Geometry check sheet. Reference: the model listing, model coordinates, mm. A direction names the side the tool comes from. Give positions to 0.01 mm unless a question says otherwise; leave off trailing zeros. Write each loop counter-clockwise with the first axis right and the second up, starting at its lowest first coordinate (ties: lowest second). Pieces come first, ordered by that corner, then holes. Notation, with made-up numbers: (85.25, -27.5) - (134.25, -27.5) arc R24 ccw to (134.25, -4.5) - close; hole circle Ø6 at (36, 1). An arc over 180 degrees is marked (long way). Write item = value, one per line. Start each with the question number.
(1) Section check B-B, the plane x = 0. Enter the section's corners in (y, z).
(2) Section check A-A, the plane y = 0. Enter the section's corners in (x, z), plus the area to 3 significant figures.
(3) Access from +Z, -Z, +X, -X, +Y, -Y to the whole of each face (thin tool, end or side, straight path). Record for faces 1 (the cylindrical face through (15.48, 11.37, 4.44)), 2 (the flat face through (24.21, -6.415, 4.437)).
(4) Section check C-C, the plane z = 5.5. Enter the section's corners in (x, y), plus the area to 3 significant figures.
(5) Draft check along Y on faces 3 (the flat face through (16, -5.139, 4)), 4 (the cylindrical face through (14.09, 7.79, 4.44)), 5 (the cylindrical face through (14.09, 2.65, 4.56)), 6 (the flat face through (15, 0, 9)). Enter one of: pulls with the +Y half, pulls with the -Y half, needs draft (parallel to the pull), parting line crosses it, or undercut.
(6) Depth check by flat-ended pin: pin 1 Ø2 at (y, z) = (6.5, 7) entering from -X; pin 2 Ø1.8 at (x, y) = (15.59, 2.59) entering from -Z; pin 3 Ø4 at (x, z) = (8.5, 2.5) entering from +Y; pin 4 Ø2 at (y, z) = (-2.5, 1) entering from +X. Enter the tip coordinate at first touch or a pass-through.
(7) Thickness scan on L1, parallel to Y at x = 0, z = 2.75; L2, parallel to X at y = 1.75, z = 6; L3, parallel to Y at x = 12.5, z = 1.25. Record the ranges inside material, lowest first.
(8) Section check D-D, the plane y = 8.5. Enter the section's corners in (x, z).
Autodesk Inventor part; units mm, degrees
ref_plane "YZ Plane" through (0, 0, 0) normal (1, 0, 0) x (0, 1, 0)
ref_plane "XZ Plane" through (0, 0, 0) normal (0, 1, 0) x (-1, 0, 0)
ref_plane "XY Plane" through (0, 0, 0) normal (0, 0, 1) x (1, 0, 0)
sketch "Sketch1" plane through (0, 0, 0) normal (0, 0, 1) x (1, 0, 0)
  line L0 (19.4476, -5.1392) -> (29.1069, -7.7274)
  line L1 (19.4476, -5.1392) -> (23.5887, 10.3156) construction
  line L2 (11.7298, -5.1392) -> (19.4476, -5.1392)
  line L3 (7.5887, 10.3156) -> (11.7298, -5.1392) construction
  line L4 (7.5887, 10.3156) -> (23.5887, 10.3156) construction
  arc A0 (23.5887, 10.3156) -> (7.5887, 10.3156) centre (15.5887, -19.5408) ccw
  line L5 (11.7298, -5.1392) -> (2.0706, -7.7274)
  line L6 (-2.0706, 7.7274) -> (7.5887, 10.3156)
  arc A1 (-2.0706, 7.7274) -> (2.0706, -7.7274) centre (0, 0) ccw
  circle A2 centre (0, 0) radius 8 construction
  circle A3 centre (31.1774, 0) radius 8 construction
  arc A4 (29.1069, -7.7274) -> (33.248, 7.7274) centre (31.1774, 0) ccw
  line L7 (23.5887, 10.3156) -> (33.248, 7.7274)
  circle A5 centre (0, 0) radius 1.5
  circle A6 centre (31.1774, 0) radius 1.5
  circle A7 centre (15.5887, 7.8608) radius 1.5
  point P0 (0, 0)
  point P1 (15.5887, 10.3156)
  dimension "d0" = 16
  dimension "d1" = 16
  dimension "d2" = 16
  dimension "d3" = 10
  dimension "d4" = 10
  dimension "d5" = 16
  dimension "d6" = 16
  dimension "d7" = 75
  dimension "d8" = 3
  dimension "d9" = 3
  dimension "d10" = 3
  dimension "d11" = 13
extrude "Extrusion1" add sketch "Sketch1" along normal blind 9
sketch "Sketch3" plane through (0, 0, 9) normal (0, 0, 1) x (1, 0, 0)
  circle A0 centre (15.5887, 2.5882) radius 1.5
  line L0 (11.7298, -5.1392) -> (19.4476, -5.1392) construction
  line L1 (7.5887, 10.3156) -> (-2.0706, 7.7274) construction
  line L2 (33.248, 7.7274) -> (23.5887, 10.3156) construction
  line L3 (7.5887, 10.3156) -> (23.5887, 10.3156) construction
  line L4 (15.5887, 10.3156) -> (15.5887, -5.1392) construction
  point P0 (0, 0)
  point P1 (15.5887, 2.5882)
  dimension "d19" = 3
extrude "Extrusion3" cut sketch "Sketch3" against normal through all
properties material "ABS Plastic"
Model answer:
q1.outline = (-8, 0) - (-1.5, 0) - (-1.5, 9) - (-8, 9) - close; (1.5, 0) - (8.28, 0) - (8.28, 9) - (1.5, 9) - close
q2.outline = (-8, 0) - (-1.5, 0) - (-1.5, 9) - (-8, 9) - close; (1.5, 0) - (29.68, 0) - (29.68, 9) - (1.5, 9) - close; (32.68, 0) - (39.18, 0) - (39.18, 9) - (32.68, 9) - close
q2.area = 371 mm²
q3.face_1 = +Z, -Z, +Y
q3.face_2 = +Z, -Z, -Y
q4.outline = (-2.07, 7.73) arc R8 ccw to (2.07, -7.73) - (11.73, -5.14) - (19.45, -5.14) - (29.11, -7.73) arc R8 ccw to (33.25, 7.73) - (23.59, 10.32) arc R30.91 ccw to (7.59, 10.32) - close; hole circle Ø3 at (0, 0); hole circle Ø3 at (15.59, 2.59); hole circle Ø3 at (15.59, 7.86); hole circle Ø3 at (31.18, 0)
q4.area = 687 mm²
q5.face_3 = pulls with the -Y half
q5.face_4 = undercut
q5.face_5 = undercut
q5.face_6 = needs draft
q6.pin_1 = -5.81
q6.pin_2 = through
q6.pin_3 = 10.95
q6.pin_4 = 39.04
q7.L1 = -8 to -1.5, 1.5 to 8.28
q7.L2 = -7.81 to 14.34, 16.83 to 38.98
q7.L3 = -5.14 to 11.21
q8.outline = (0.81, 0) - (14.23, 0) - (14.23, 9) - (0.81, 9) - close; (16.95, 0) - (30.36, 0) - (30.36, 9) - (16.95, 9) - close
